Source: three-view drawing plus pictorial views. Frame: mm from the lowest corner of the part. A direction names the side the tool comes from. Give positions to 0.01 mm unless a question says otherwise; leave off trailing zeros. Order: outer loops, then holes, each group sorted by start corner. A loop starts at its lowest first (then second) coordinate and runs counter-clockwise, first axis right, second up. Notation, with made-up numbers: (78, 55) - (127, 55) arc R21 cw to (127, 62) - close; hole circle Ø7 at (31.25, 58.5). An arc over 180 degrees is marked (long way). Answer in a Markdown table with one row per item. Add a question column.
1. Contact query for a flat-ended pin moving along its axis: pin 1 (3 mm diameter, centred on x = 151, z = 59, fed in from +Y). Output: stop coordinate, or through.
2. Section query B-B on z = 84. Return loops of the section in (x, y).
3. Access query for the marked faces 1, 2 and 3. Directions: +Z, -Z, +X, -X, +Y, -Y. A direction counts if a zero-diameter tool reaches every point of the face in a straight line with its end or side. Return the directions, or none.
4. Section query C-C on y = 99. Return loops of the section in (x, z), and give its area (3 significant figures).
5. Mould query, pull axis Z, two halves, no side actions, for the marked faces 4, 5, 6 and 7. Classes: released by +Z, released by -Z, zero draft, split by the parting line, or undercut.
6. Ray query, line 1 (X direction, y = 112, z = 85.5); line 2 (Y direction, x = 104, z = 133). Return the intervals inside material, ascending. Write a range as [from, to].
7. Section query D-D on x = 85. Return loops of the section in (y, z).
8. Section query A-A on x = 146.5. Return loops of the section in (y, z).
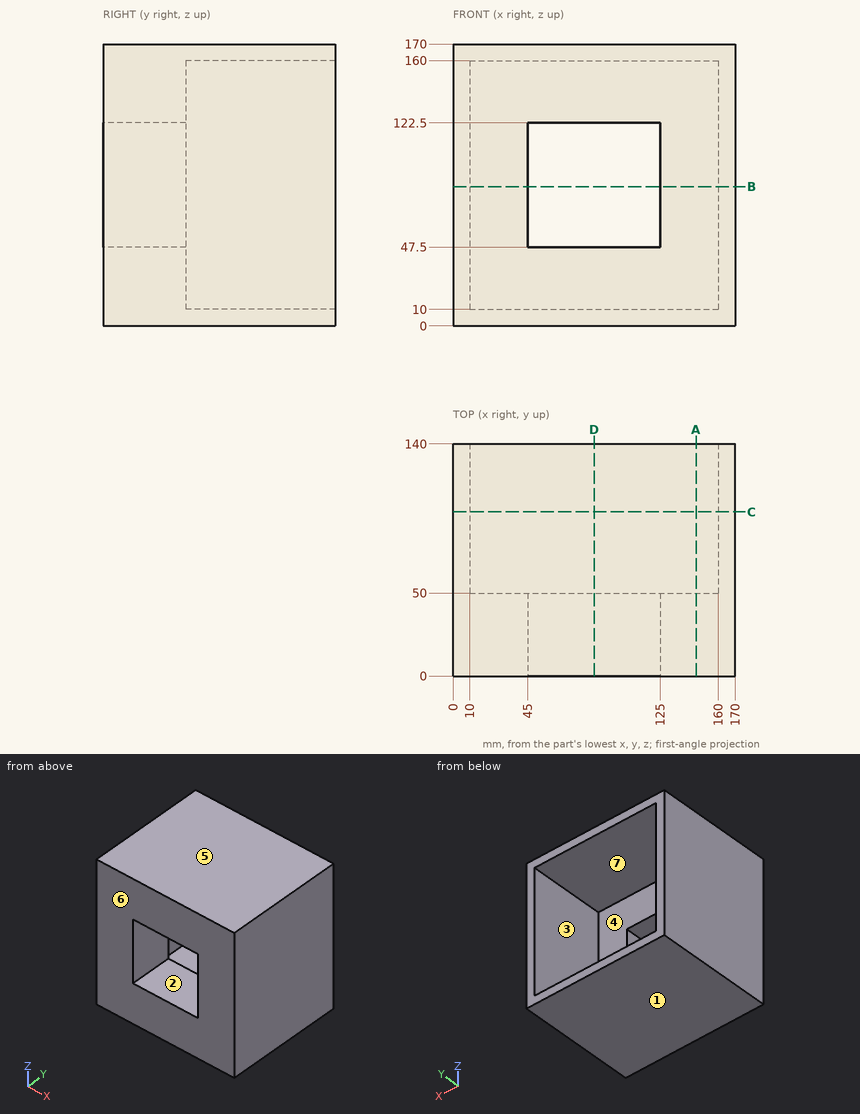
Answer:
| question | item | result |
|---|---|---|
| 1 | pin 1 | stops at y = 50 |
| 2 | outline | (0, 0) - (45, 0) - (45, 50) - (10, 50) - (10, 140) - (0, 140) - close; (125, 0) - (170, 0) - (170, 140) - (160, 140) - (160, 50) - (125, 50) - close |
| 3 | face 1 | -Z, +X, -X, +Y, -Y |
| 3 | face 2 | +Y, -Y |
| 3 | face 3 | +Y |
| 4 | outline | (0, 0) - (170, 0) - (170, 170) - (0, 170) - close; hole (10, 10) - (160, 10) - (160, 160) - (10, 160) - close |
| 4 | area | 6,400 mm² |
| 5 | face 4 | undercut |
| 5 | face 5 | released by +Z |
| 5 | face 6 | zero draft |
| 5 | face 7 | undercut |
| 6 | line 1 | x = [0, 10], [160, 170] |
| 6 | line 2 | y = [0, 50] |
| 7 | outline | (0, 0) - (140, 0) - (140, 10) - (50, 10) - (50, 47.5) - (0, 47.5) - close; (0, 122.5) - (50, 122.5) - (50, 160) - (140, 160) - (140, 170) - (0, 170) - close |
| 8 | outline | (0, 0) - (140, 0) - (140, 10) - (50, 10) - (50, 160) - (140, 160) - (140, 170) - (0, 170) - close |
